Source: CAD feature listing. Evaluate the final solid. Frame: model axes, mm. A direction names the side the tool comes from. Round coordinates to 2 decimals unless told otherwise and drop trailing zeros. Write each loop counter-clockwise with the first axis right and the second up, starting at its lowest first coordinate (ties: lowest second). Pieces come first, ordered by that corner, then holes. Notation, with made-up numbers: M -7,17 L -3,17 A10 cw -3,29 Z; hole C 83,-2 d2. An arc over 180 degrees is marked long. Answer in a Markdown table with one row per item. Add a question column.
Item 1: Material intervals for probe 1 along Y at (x, z) = (54.5, 3.25); probe 2 along X at (y, z) = (-50, 2) (3 decimals); probe 3 along X at (y, z) = (-1, 4.25), sorted ascending.
Item 2: Mould query, pull axis X, two halves, no side actions, for faces 1 (the face through (-2, 1, 0)), 2 (the face through (-41.51, -43.92, 9.74)), 3 (the face through (115, -1, 6)). Classes: released by +X, released by -X, zero draft, split by the parting line, or undercut.
Item 3: Set-up query: faces 4 (the face through (-36.826, 51.214, 9.742)), 5 (the face through (-1.33, 23.48, 3.3)). Return all of +Z, -Z, +X, -X, +Y, -Y with unobstructed straight access to the full face (end or side cutting, diameter ignored); none if empty.
Item 4: Cut plane A-A on x = -1. Return loops of the section in (y, z).
Item 5: Cut plane C-C on z = 10.25. Return loops of the section in (x, y) (3 decimals).
Item 6: Cut plane B-B on y = -1. Return loops of the section in (x, z).
Item 7: Contact query for flat-ended pins moving along their axis: pin 1 (8 mm diameter, centred on x = 21, y = -1, fed in from +Z); pin 2 (5.5 mm diameter, centred on x = -34.875, y = 60, fed in from +Z). Output: stop coordinate, or through.
Item 8: Cut plane D-D on y = 60. Return loops of the section in (x, z) (3 decimals), and give its area (3 significant figures).
from build123d import *

# Parameters (mm, degrees)
F0_W     = 230
F0_H     = 180
F0_R     = 3.56
F0_R_2   = 2.5
F1_DEPTH = 12.7
F2_R     = 9
F2_R_2   = 5
F3_DEPTH = 6


# Not quite as in the source:
# - a length typed as a fraction of an inch, garbled in the dataset ("3 / 203.2 mm" for 3/8 in), is restored


with BuildPart() as f1:
    # F0 (on Top) → F1 (new body)
    with BuildSketch(Plane.XY):
        Rectangle(F0_W, F0_H)
        with Locations((-34.875, -50)):
            Circle(F0_R, mode=Mode.SUBTRACT)
        with Locations((54.875, -50)):
            Circle(F0_R_2, mode=Mode.SUBTRACT)
        with Locations((21, -1)):
            Circle(F0_R_2, mode=Mode.SUBTRACT)
        with Locations((-1, 21)):
            Circle(F0_R_2, mode=Mode.SUBTRACT)
        with Locations((-34.875, 60)):
            Circle(F0_R, mode=Mode.SUBTRACT)
        with Locations((54.875, 60)):
            Circle(F0_R_2, mode=Mode.SUBTRACT)
    extrude(amount=F1_DEPTH)

    # F2 (on face) → F3 (cut)
    with BuildSketch(Plane.XY.offset(12.7)):
        with Locations((-34.875, 60)):
            Circle(F2_R)
        with Locations((54.875, 60)):
            Circle(F2_R)
        with Locations((-34.875, -50)):
            Circle(F2_R)
        with Locations((54.875, -50)):
            Circle(F2_R)
        with Locations((-1, 21)):
            Circle(F2_R_2)
        with Locations((21, -1)):
            Circle(F2_R_2)
    extrude(amount=-F3_DEPTH, mode=Mode.SUBTRACT)


solid = f1.part
Results below:
| question | item | result |
|---|---|---|
| 1 | probe 1 | -90 to -52.47, -47.53 to 57.53, 62.47 to 90 |
| 1 | probe 2 | -115 to -38.435, -31.315 to 52.375, 57.375 to 115 |
| 1 | probe 3 | -115 to 18.5, 23.5 to 115 |
| 2 | face 1 | zero draft |
| 2 | face 2 | undercut |
| 2 | face 3 | released by +X |
| 3 | face 4 | +Z |
| 3 | face 5 | +Z, -Z |
| 4 | outline | M -90,0 L 18.5,0 L 18.5,6.7 L 16,6.7 L 16,12.7 L -90,12.7 Z; M 23.5,0 L 90,0 L 90,12.7 L 26,12.7 L 26,6.7 L 23.5,6.7 Z |
| 5 | outline | M -115,-90 L 115,-90 L 115,90 L -115,90 Z; hole C -34.875,-50 d18; hole C -34.875,60 d18; hole C -1,21 d10; hole C 21,-1 d10; hole C 54.875,-50 d18; hole C 54.875,60 d18 |
| 6 | outline | M -115,0 L 18.5,0 L 18.5,6.7 L 16,6.7 L 16,12.7 L -115,12.7 Z; M 23.5,0 L 115,0 L 115,12.7 L 26,12.7 L 26,6.7 L 23.5,6.7 Z |
| 7 | pin 1 | z = 6.7 |
| 7 | pin 2 | through |
| 8 | outline | M -115,0 L -38.435,0 L -38.435,6.7 L -43.875,6.7 L -43.875,12.7 L -115,12.7 Z; M -31.315,0 L 52.375,0 L 52.375,6.7 L 45.875,6.7 L 45.875,12.7 L -25.875,12.7 L -25.875,6.7 L -31.315,6.7 Z; M 57.375,0 L 115,0 L 115,12.7 L 63.875,12.7 L 63.875,6.7 L 57.375,6.7 Z |
| 8 | area | 2,620 mm2 |
